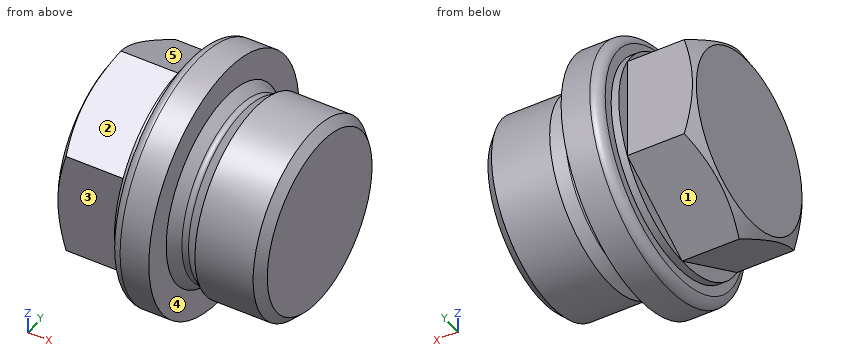
Autodesk Inventor part; units mm, degrees
ref_plane "YZ Plane" through (0, 0, 0) normal (1, 0, 0) x (0, 1, 0)
ref_plane "XZ Plane" through (0, 0, 0) normal (0, 1, 0) x (-1, 0, 0)
ref_plane "XY Plane" through (0, 0, 0) normal (0, 0, 1) x (1, 0, 0)
sketch "Эскиз1" plane through (0, 0, 0) normal (0, 0, 1) x (1, 0, 0)
  line L0 (10, 0) -> (10, 10)
  line L1 (10, 10) -> (3, 10)
  line L2 (3, 10) -> (1.8448, 9.1888)
  line L3 (1.1552, 9.1888) -> (0, 10)
  line L4 (0, 10) -> (0, 13)
  line L5 (0, 13) -> (-4, 13)
  line L6 (-4, 13) -> (-4, 10.9697)
  line L7 (-4, 10.9697) -> (-4.8, 10.9697)
  line L8 (-4.8, 10.9697) -> (-4.8, 0)
  line L9 (-4.8, 0) -> (10, 0)
  arc A0 (1.1552, 9.1888) -> (1.8448, 9.1888) centre (1.5, 9.6798) ccw
  line L10 (-7.8876, 0) -> (13.7255, 0)
  line L11 (0, -2.6) -> (0, 15.6)
  line L12 (2.3733, 9.0798) -> (10.6379, 9.0798) construction
  dimension "d0" = 0.6
  dimension "d1" = 20
  dimension "d2" = 26
  dimension "d3" = 10
  dimension "d4" = 3
  dimension "d5" = 1.5
  dimension "d6" = 21.9393
  dimension "d7" = 4
  dimension "d8" = 0.8
  dimension "d10" = 18.1596
revolve "Базовый элемент" add sketch "Эскиз1" angle 360 about axis through (-4.8, 0, 0) along (1, 0, 0)
sketch "Эскиз2" plane through (-4.8, 0, 0) normal (-1, 0, 0) x (0, 0, 1)
  circle A0 centre (0, 0) radius 10.9697
  line L0 (10.9697, 0) -> (5.4848, -9.5)
  line L1 (5.4848, -9.5) -> (-5.4848, -9.5)
  line L2 (-5.4848, -9.5) -> (-10.9697, 0)
  line L3 (-10.9697, 0) -> (-5.4848, 9.5)
  line L4 (-5.4848, 9.5) -> (5.4848, 9.5)
  line L5 (5.4848, 9.5) -> (10.9697, 0)
extrude "С головкой" add sketch "Эскиз2" along normal blind 7 contours L0 L1 L2 L3 L4 L5
fillet "Сопряжение1" radius 1 1 edges at (-4, -13, 0)
sketch "Эскиз3" plane through (0, 0, 0) normal (0, 1, 0) x (-1, 0, 0)
  line L0 (10.75, 10.9697) -> (11.8, 9.151)
  line L1 (11.8, 9.151) -> (11.8, 10.9697)
  line L2 (11.8, 10.9697) -> (10.75, 10.9697)
  line L3 (12.01, 0) -> (10.54, 0)
  dimension "d14" = 1.05
  dimension "d15" = 30
revolve "Фаска1" cut sketch "Эскиз3" angle 360 about axis through (-10, 0, 0) along (1, 0, 0)
thread "Резьба1"
chamfer "Фаска2" distance 0.9202 distance2 0.9202 1 edges at (10, -10, 0) measured on face at (7.6667, 9.9676, -0.8047)
equation "\"d12\" = KOH"
equation "\"d14\" = 0.15 * KOH"
equation "\"d17\" = RR"
equation "\"d20\" = NLG"
equation "\"d18\" = GAL"
equation "\"d19\" = -0.5 * GD1 + 0.5 * NND"
equation "\"d0\" = 0.2 * GAL1"
equation "\"d1\" = NND"
equation "\"d2\" = KOD"
equation "\"d3\" = NLG"
equation "\"d4\" = GAL1"
equation "\"d5\" = 0.5 * GAL1"
equation "\"d6\" = n_D"
equation "\"d7\" = SD"
equation "\"d8\" = PHH"
equation "\"d10\" = GD1"
equation "\"NLG\" = 10"
equation "\"NND\" = 20"
equation "\"SD\" = 4"
equation "\"PHH\" = 0.8"
equation "\"SW\" = 19"
equation "\"GAL1\" = 3"
equation "\"KOH\" = 7"
equation "\"KOD\" = 26"
equation "\"GAL\" = 0.61345 * PTC"
equation "\"RR\" = 1"
equation "\"GD1\" = THREADDIA - 1.2269 * PTC"
equation "\"n_D\" = 1.1547 * SW"
equation "\"GUL\" = 0.61345 * PTC"
equation "\"TOA\" = 30deg"
equation "\"PTC\" = 1.5"
properties part number "CSN 02 1915.21 - M 20 x 10" material "Сталь, мягкая"
Input: part model. Units: mm. Frame: model coordinates. Face numbers are marked on the shaded views. A direction names the side the tool comes from. Round coordinates to 2 decimals unless told otherwise and drop trailing zeros. Loops run counter-clockwise (first coordinate to the right, second up) from the corner with the lowest first, then second, coordinate; pieces in that order, holes last. Notation, with made-up numbers: M 86.25,52 L 92.25,52 A11 cw 92.25,69 Z; hole C 75.5,53 d11. An arc over 180 degrees is marked long. Answer in a Markdown table with one row per item. Add a question column.
1. Section B-B (x = -8.5). Output: boundary loops of the cut face in (y, z).
2. Section C-C (x = 6.25). Output: boundary loops of the cut face in (y, z).
3. Section D-D (x = 0.5). Output: boundary loops of the cut face in (y, z), and give its area (3 significant figures).
4. Ray query, probe 1 along Y at (x, z) = (-0.5, 0.25); probe 2 along X at (y, z) = (7, 9); probe 3 along Y at (x, z) = (-5, 2). Return the intervals inside material, ascending.
5. Set-up query: the marked faces 1, 2, 3, 4 and 5. Return all of +Z, -Z, +X, -X, +Y, -Y with unobstructed straight access to the full face (end or side cutting, diameter ignored); none if empty.
6. Contact query for flat-ended pins moving along their axis: pin 1 (7.5 mm diameter, centred on x = -9.5, z = -1.5, fed in from -Y); pin 2 (1.6 mm diameter, centred on y = -10, z = -1, fed in from -X); pin 3 (4 mm diameter, centred on x = -5.5, z = -5.5, fed in from -Y). Output: stop coordinate, or through.
7. Section A-A (z = 0). Output: boundary loops of the cut face in (x, y).
Values follow:
| question | item | result |
|---|---|---|
| 1 | outline | M -9.5,-5.48 L 0,-10.97 L 9.5,-5.48 L 9.5,5.48 L 0,10.97 L -9.5,5.48 Z |
| 2 | outline | C 0,0 d20 |
| 3 | outline | C 0,0 d19.3 |
| 3 | area | 292 mm^2 |
| 4 | probe 1 | -13 to 13 |
| 4 | probe 2 | -4 to 0 |
| 4 | probe 3 | -9.5 to 9.5 |
| 5 | face 1 | -Z, -X, +Y |
| 5 | face 2 | +Z, -X, -Y |
| 5 | face 3 | +Z, -Z, -X, -Y |
| 5 | face 4 | +X |
| 5 | face 5 | +Z, -X, +Y |
| 6 | pin 1 | y = -9.5 |
| 6 | pin 2 | x = -11.74 |
| 6 | pin 3 | y = -11.85 |
| 7 | outline | M -11.8,-9.15 L -11.6,-9.5 L -4.8,-9.5 L -4.8,-10.97 L -4,-10.97 L -4,-12 A1 ccw -3,-13 L 0,-13 L 0,-10 L 1.16,-9.19 A0.6 cw 1.84,-9.19 L 3,-10 L 9.08,-10 L 10,-9.08 L 10,9.08 L 9.08,10 L 3,10 L 1.84,9.19 A0.6 cw 1.16,9.19 L 0,10 L 0,13 L -3,13 A1 ccw -4,12 L -4,10.97 L -4.8,10.97 L -4.8,9.5 L -11.6,9.5 L -11.8,9.15 Z |
